CAD build for the part. Positions are in the model's coordinates, mm. A direction names the side the tool comes from. Round coordinates to 2 decimals unless told otherwise and drop trailing zeros. Order: outer loops, then holes, each group sorted by start corner. A loop starts at its lowest first (then second) coordinate and runs counter-clockwise, first axis right, second up.
```python
from build123d import *

# Parameters (mm, degrees)
SKETCH1_R           = 2.95
BOSS_EXTRUDE1_DEPTH = 2.5
SKETCH2_R           = 1.5
BOSS_EXTRUDE2_DEPTH = 20
CHAMFER1_SIZE       = 0.3
CUT_EXTRUDE1_DEPTH  = 2
FILLET1_R           = 1


with BuildPart() as part:
    # Sketch1 → Boss-Extrude1 (new body)
    with BuildSketch(Plane.XY):
        Circle(SKETCH1_R)
    extrude(amount=BOSS_EXTRUDE1_DEPTH)

    # Sketch2 → Boss-Extrude2 (add)
    with BuildSketch(Plane(origin=(0, 0, 0), x_dir=(-1, 0, 0), z_dir=(0, 0, -1))):
        with Locations(Location((0, 0, 0), (0, 0, 180))):
            Circle(SKETCH2_R)
    extrude(amount=BOSS_EXTRUDE2_DEPTH)

    # Chamfer1
    chamfer1_edges = [part.edges().sort_by_distance(p)[0] for p in [
        (-1.5, 0, -20),
    ]]
    chamfer(chamfer1_edges, length=CHAMFER1_SIZE)

    # Sketch3 → Cut-Extrude1 (cut)
    with BuildSketch(Plane.XY.offset(2.5)):
        Polygon((0.363589324, 0.363589324), (2, 0.363589324), (2, -0.363589324), (0.363589324, -0.363589324), (0.363589324, -2), (-0.363589324, -2), (-0.363589324, -0.363589324), (-2, -0.363589324), (-2, 0.363589324), (-0.363589324, 0.363589324), (-0.363589324, 2), (0.363589324, 2), align=None)
    extrude(amount=-CUT_EXTRUDE1_DEPTH, mode=Mode.SUBTRACT)

    # Fillet1
    # the kernel refuses this fillet: 1 mm, written as the material it takes off along each edge
    with BuildSketch(Plane(origin=(0, 0, 2.5), x_dir=(1, 0, 0), z_dir=(0, -1, 0))) as fillet1_piece_1:
        with BuildLine():
            CenterArc((2.95 - FILLET1_R, -FILLET1_R), FILLET1_R, 0, 90)
            Line((2.95 - FILLET1_R, 0), (2.95, 0))
            Line((2.95, 0), (2.95, -FILLET1_R))
        make_face()
    revolve(axis=Axis((0, 0, 2.5), (0, 0, 1)), mode=Mode.SUBTRACT)


solid = part.part
```
1. Pin check, flat tips, straight feed: P1, Ø0.8, axis at y = 1, z = 1.5, coming from the -X side; P2, Ø1.8, axis at x = 1.5, z = 1.5, coming from the -Y side; P3, Ø1.5, axis at x = 2, z = -11.5, coming from the -Y side. Stop position of each tip, or through.
2. Drill centre lines: line 1 (X direction, y = 0.1, z = -11.75); line 2 (Z direction, x = 0.2, y = 0.3); line 3 (Z direction, x = 0.9, y = 1.45). Where is each one in solid material? Low to high.
3. Tool access for faces 1 (the face through (1.43, -0.45, -9.71)), 2 (the face through (1, 1, 2.5)), 3 (the face through (-1, 0.364, 2)): list every direction of +Z, -Z, +X, -X, +Y, -Y with a clear straight run to the whole face (end or side of a thin tool).
4. Cut at C-C, the plane z = -18.25. Write the cut outline in (x, y), and give its area (3 significant figures).
5. Cut at A-A, the plane x = 0. Write the cut outline in (y, z).
6. Mould opens along Y. For faces 4 (the face through (-1, 1, 2.5)), 5 (the face through (0.364, 1, 2)), 6 (the face through (-2.947, 0.13, 0.74)) say: released by +Y, released by -Y, zero draft, split by the parting line, or undercut.
Outcome:
1. P1: stops at x = -2.89
1. P2: stops at y = -2.89
1. P3: stops at y = -0.83
2. line 1: x = -1.5 to 1.5
2. line 2: z = -20 to 0.5
2. line 3: z = 0 to 2.5
3. face 1: -Z
3. face 2: +Z, +X, -X, +Y, -Y
3. face 3: +Z
4. outline: circle Ø3 at (0, 0)
4. area: 7.07 mm2
5. outline: (-2.95, 0) - (-1.5, 0) - (-1.5, -19.7) - (-1.2, -20) - (1.2, -20) - (1.5, -19.7) - (1.5, 0) - (2.95, 0) - (2.95, 1.5) arc R1 ccw to (2, 2.5) - (2, 0.5) - (-2, 0.5) - (-2, 2.5) arc R1 ccw to (-2.95, 1.5) - close
6. face 4: zero draft
6. face 5: undercut
6. face 6: split by the parting line
